Study the drawing (mm; zero at the part's minimum x, y, z) and answer. A direction names the side the tool comes from. Round coordinates to 2 decimals unless told otherwise and drop trailing zeros. Order: outer loops, then holes, each group sorted by start corner. A loop starts at its lowest first (then second) coordinate and runs counter-clockwise, first axis right, second up. Notation, with made-up numbers: (39, 55.25) - (51, 55.25) arc R24 ccw to (51, 72.25) - close; hole circle Ø1 at (57.25, 42). An arc over 180 degrees is marked (long way). Put each result on its own line as item: value. Start each with the question number.
Q1. Section B-B on z = 1 is taken. Give the vertices of the cut face in (x, y).
Q2. Which of the six approach directions +Z, -Z, +X, -X, +Y, -Y give full straight-line access (tool end or side, diameter ignored) to the marked faces 1, 2 and 3?
Q3. Section A-A on y = 4 is taken. Give the vertices of the cut face in (x, z) (1 decimal).
Q4. Each of these flat-tipped pins is pushed along its axis until it touches: pin 1 Ø1.5 at (y, z) = (26, 2) entering from +X (1 decimal); pin 2 Ø3 at (x, z) = (87.55, 4.78) entering from +Y; pin 3 Ø5 at (x, z) = (89, 3) entering from +Y; pin 4 Ø4 at (x, z) = (40.5, 2) entering from +Y. Where does it stop, or does it pass through?
Q5. Section D-D on x = 76 is taken. Give the vertices of the cut face in (y, z), then the cut area to 3 significant figures.
Q6. Section C-C on y = 24 is taken. Give the vertices of the cut face in (x, z) (1 decimal), then the cut area to 3 significant figures.
Q7. Find the intervals of material crossed by line 1 along Y through (x, z) = (90, 3.5); line 2 along X through (y, z) = (17.5, 1.75) (1 decimal); line 3 along X through (y, z) = (7, 5.25), in increasing order. Write a range as from..to.
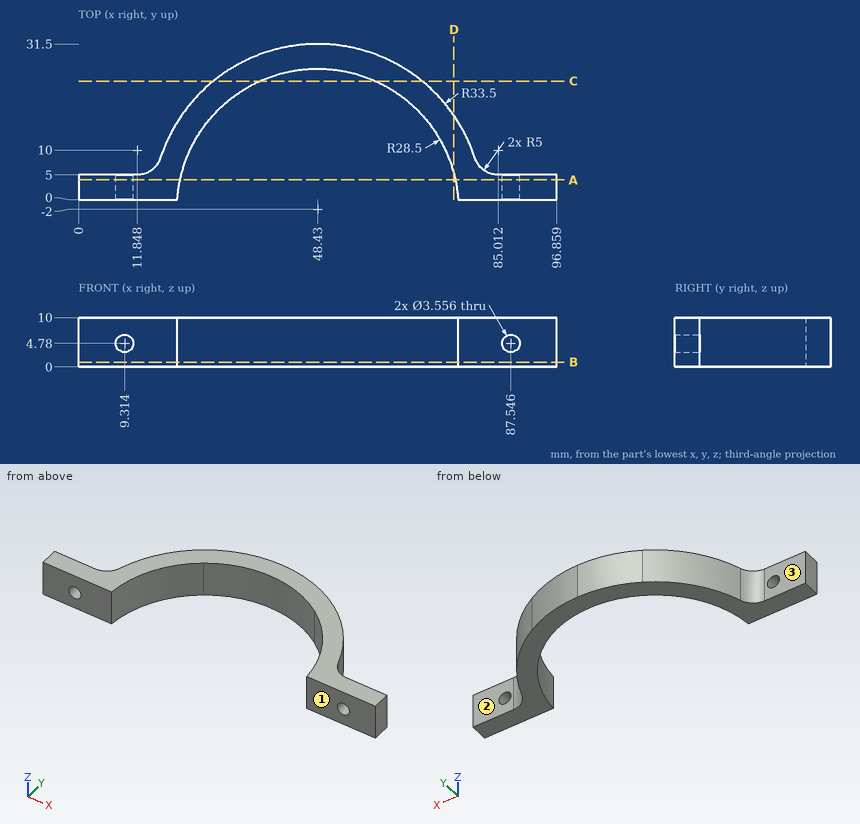
Findings:
1. outline: (0, 0) - (20, 0) arc R28.5 cw to (76.86, 0) - (96.86, 0) - (96.86, 5) - (85.01, 5) arc R5 cw to (80.26, 8.44) arc R33.5 ccw to (16.6, 8.44) arc R5 cw to (11.85, 5) - (0, 5) - close
2. face 1: +Z, -Z, +X, -X, -Y
2. face 2: +Z, -Z, +X, +Y
2. face 3: +Z, -Z, -X, +Y
3. outline: (0, 0) - (20.6, 0) - (20.6, 10) - (0, 10) - close; (76.3, 0) - (96.9, 0) - (96.9, 10) - (76.3, 10) - close; hole circle Ø3.6 at (9.3, 4.8); hole circle Ø3.6 at (87.5, 4.8)
4. pin 1: x = 67.9
4. pin 2: through
4. pin 3: y = 5
4. pin 4: y = 30.97
5. outline: (5.22, 0) - (17.03, 0) - (17.03, 10) - (5.22, 10) - close
5. area: 118 mm2
6. outline: (27.3, 0) - (36.8, 0) - (36.8, 10) - (27.3, 10) - close; (60.1, 0) - (69.6, 0) - (69.6, 10) - (60.1, 10) - close
6. area: 189 mm2
7. line 1: 0..5
7. line 2: 21.2..27.6, 69.2..75.7
7. line 3: 15.85..21.39, 75.47..81.01
